Here's how the part is built. I have some questions about the finished solid (model axes, mm). Face numbers are marked on the shaded views. Round coordinates to 2 decimals unless told otherwise and drop trailing zeros. Loops run counter-clockwise (first coordinate to the right, second up) from the corner with the lowest first, then second, coordinate; pieces in that order, holes last. Notation, with made-up numbers: (4, 89) - (47, 89) arc R23 ccw to (47, 121) - close; hole circle Ø1 at (13.25, 56). An arc over 180 degrees is marked (long way). Answer as a JSON object with one key per item and string values. Group by question number.
1) I want a section at A-A, the plane y = 0. Please give me the cut outline in (x, z).
2) If we mould it in two halves opening along X, with no side actions, what happens to the marked faces 1, 2, 3 and 4? For each: pulls with the +X half, pulls with the -X half, needs draft (parallel to the pull), parting line crosses it, or undercut.
3) I want a section at D-D, the plane y = -5.5. Please give me the cut outline in (x, z), then the cut area to 3 significant figures.
4) Will these pins go through, and if not, where does the flat tip stop? P1, Ø4, axis at y = -9, z = 16.5, coming from the +X side (3 decimals); P2, Ø1.5, axis at y = -12, z = 16.5, coming from the +X side; P3, Ø17, axis at x = 0, y = 0, coming from the +Z side.
5) I want a section at B-B, the plane x = 0. Please give me the cut outline in (y, z), then the cut area to 3 significant figures.
6) I want a section at C-C, the plane z = 2. Please give me the cut outline in (x, y).
7) If I drill on line 1 along X through (y, z) = (0, 5.25); line 2 along X through (y, z) = (-9, 10.5); line 3 along Y through (x, z) = (0, 13), over which ranges is the centre line in solid material (lowest first)? Write a range as [from, to].
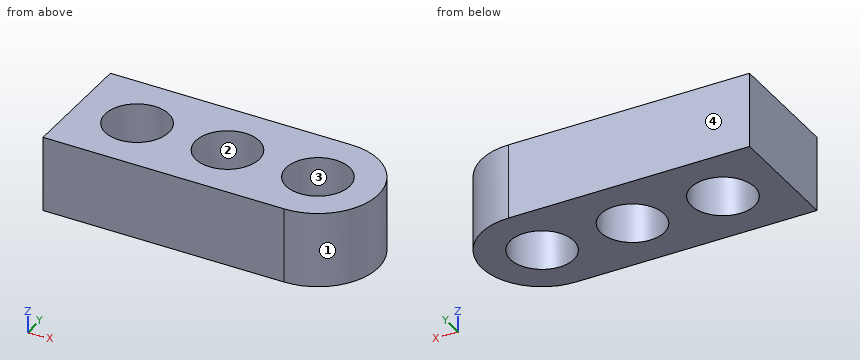
from build123d import *

# Parameters (mm, degrees)
F0_W     = 80
F0_H     = 40
F1_DEPTH = 25
F2_R     = 10.527281
F3_DEPTH = 25


with BuildPart() as f1:
    # F0 (on Top) → F1 (new body)
    with BuildSketch(Plane.XY):
        with Locations((-10, 0)):
            Rectangle(F0_W, F0_H)
        with BuildLine():
            ThreePointArc((30, -20), (50, 0), (30, 20))
            Line((30, 20), (30, -20))
        make_face()
    extrude(amount=F1_DEPTH)

    # F2 (on face) → F3 (cut, through all)
    with BuildSketch(Plane(origin=(0, 0, 0), x_dir=(1, 0, 0), z_dir=(0, 0, -1))):
        with Locations((30, 0)):
            Circle(F2_R)
        Circle(F2_R)
        with Locations((-30, 0)):
            Circle(F2_R)
    extrude(amount=-F3_DEPTH, mode=Mode.SUBTRACT)


solid = f1.part
Outcome:
{
 "1": {"outline": "(-50, 0) - (-40.53, 0) - (-40.53, 25) - (-50, 25) - close; (-19.47, 0) - (-10.53, 0) - (-10.53, 25) - (-19.47, 25) - close; (10.53, 0) - (19.47, 0) - (19.47, 25) - (10.53, 25) - close; (40.53, 0) - (50, 0) - (50, 25) - (40.53, 25) - close"},
 "2": {"face 1": "pulls with the +X half", "face 2": "undercut", "face 3": "undercut", "face 4": "needs draft"},
 "3": {"outline": "(-50, 0) - (-38.98, 0) - (-38.98, 25) - (-50, 25) - close; (-21.02, 0) - (-8.98, 0) - (-8.98, 25) - (-21.02, 25) - close; (8.98, 0) - (21.02, 0) - (21.02, 25) - (8.98, 25) - close; (38.98, 0) - (49.23, 0) - (49.23, 25) - (38.98, 25) - close", "area": "1,130 mm^2"},
 "4": {"P1": "x = 48.735", "P2": "x = 46.54", "P3": "through"},
 "5": {"outline": "(-20, 0) - (-10.53, 0) - (-10.53, 25) - (-20, 25) - close; (10.53, 0) - (20, 0) - (20, 25) - (10.53, 25) - close", "area": "474 mm^2"},
 "6": {"outline": "(-50, -20) - (30, -20) arc R20 ccw to (30, 20) - (-50, 20) - close; hole circle Ø21.05 at (-30, 0); hole circle Ø21.05 at (0, 0); hole circle Ø21.05 at (30, 0)"},
 "7": {"line 1": "[-50, -40.53], [-19.47, -10.53], [10.53, 19.47], [40.53, 50]", "line 2": "[-50, -35.46], [-24.54, -5.46], [5.46, 24.54], [35.46, 47.86]", "line 3": "[-20, -10.53], [10.53, 20]"}
}
